```python
from build123d import *

# Parameters (mm, degrees)
SKETCH1_W           = 2.54
SKETCH1_H           = 2.54
BOSS_EXTRUDE1_DEPTH = 27.94
SKETCH2_W           = 0.64
SKETCH2_H           = 0.64
BOSS_EXTRUDE2_DEPTH = 6.1
LPATTERN1_COUNT     = 11
LPATTERN1_PITCH     = 2.54
SKETCH3_W           = 0.64
SKETCH3_H           = 0.64
BOSS_EXTRUDE3_DEPTH = 2.3
LPATTERN2_COUNT     = 11
LPATTERN2_PITCH     = 2.54
SKETCH4_W           = 0.64
SKETCH4_H           = 0.64
BOSS_EXTRUDE4_DEPTH = 3
LPATTERN3_COUNT     = 11
LPATTERN3_PITCH     = 2.54


with BuildPart() as part:
    # Sketch1 → Boss-Extrude1 (new body)
    with BuildSketch(Plane.XY):
        with Locations((1.27, 1.27)):
            Rectangle(SKETCH1_W, SKETCH1_H)
    extrude(amount=BOSS_EXTRUDE1_DEPTH)

    # Sketch2 → Boss-Extrude2 (add)
    with BuildSketch(Plane.XZ):
        with Locations((1.27, 26.67)):
            Rectangle(SKETCH2_W, SKETCH2_H)
    boss_extrude2 = extrude(amount=BOSS_EXTRUDE2_DEPTH)

    # LPattern1: Boss-Extrude2 ×11
    with Locations(*[(0, 0, -i * LPATTERN1_PITCH) for i in range(1, LPATTERN1_COUNT)]):
        add(boss_extrude2)

    # Sketch3 → Boss-Extrude3 (add)
    with BuildSketch(Plane(origin=(0, 2.54, 0), x_dir=(1, 0, 0), z_dir=(0, 1, 0))):
        with Locations((1.28, -1.26)):
            Rectangle(SKETCH3_W, SKETCH3_H)
    boss_extrude3 = extrude(amount=BOSS_EXTRUDE3_DEPTH)

    # LPattern2: Boss-Extrude3 ×11
    with Locations(*[(0, 0, i * LPATTERN2_PITCH) for i in range(1, LPATTERN2_COUNT)]):
        add(boss_extrude3)

    # Sketch4 → Boss-Extrude4 (add)
    with BuildSketch(Plane(origin=(1.6, 0, 0), x_dir=(0, 0, -1), z_dir=(1, 0, 0))):
        with Locations((-1.26, 4.52)):
            Rectangle(SKETCH4_W, SKETCH4_H)
    boss_extrude4 = extrude(amount=BOSS_EXTRUDE4_DEPTH)

    # LPattern3: Boss-Extrude4 ×11
    with Locations(*[(0, 0, i * LPATTERN3_PITCH) for i in range(1, LPATTERN3_COUNT)]):
        add(boss_extrude4)


solid = part.part
```
Here's how the part is built. I have some questions about the finished solid (model axes, mm). Coordinates: 2 decimals unless noted, no trailing zeros. Order: outer loops, then holes, each group sorted by start corner. A loop starts at its lowest first (then second) coordinate and runs counter-clockwise, first axis right, second up.
Item 1: If we section it at D-D, the plane y = 1.75: List the corners of the cut face in (x, z) for me.
Response values:
outline: (0, 0) - (2.54, 0) - (2.54, 27.94) - (0, 27.94) - close
Item 2: If we section it at A-A, the plane z = 23: List the corners of the cut face in (x, y) for me.
Response values:
outline: (0, 0) - (2.54, 0) - (2.54, 2.54) - (0, 2.54) - close
Item 3: Thinking about a two-plate mould opening in Z: for faces 1 (the face through (0, 1, 14)), 2 (the face through (1.9, 4.4, 26.98)), 3 (the face through (2, 0, 14)), which applies, pulls with the +Z half, pulls with the -Z half, needs draft (parallel to the pull), parting line crosses it, or undercut?
Response values:
face 1: needs draft
face 2: pulls with the +Z half
face 3: undercut
Item 4: I need wall thicknesses on probe 1 along Y at (x, z) = (0.6, 4.5); probe 2 along Y at (x, z) = (3.1, 26.5). Which ranges of each line are inside material? Lowest first, please.
Response values:
probe 1: y = 0 to 2.54
probe 2: y = 4.2 to 4.84
Item 5: I'm going to push flat-ended pins straight in: pin 1 Ø2 at (x, z) = (4, 12) entering from -Y; pin 2 Ø0.5 at (x, y) = (1.5, -4) entering from +Z; pin 3 Ø2 at (y, z) = (3, 20) entering from -X; pin 4 Ø0.7 at (x, y) = (3.5, 3) entering from -Z. Where does each tip first touch, or does it pass through?
Response values:
pin 1: stops at y = 4.2
pin 2: stops at z = 26.99
pin 3: stops at x = 0
pin 4: passes through
Item 6: If we section it at B-B, the plane x = 3.2: Give the number of separate pieces and of enclosed holes in the cut face, then the cut area to 3 significant figures.
Response values:
separate pieces: 11
enclosed holes: 0
area: 4.51 mm2
